Part print with two shaded views. Sizes in mm from the minimum x, y, z corner. A direction names the side the tool comes from. Round coordinates to 2 decimals unless told otherwise and drop trailing zeros. Order: outer loops, then holes, each group sorted by start corner. A loop starts at its lowest first (then second) coordinate and runs counter-clockwise, first axis right, second up. Notation, with made-up numbers: M 73,64.25 L 110,64.25 A17 ccw 110,81.25 Z; hole C -23.5,72 d2. An arc over 180 degrees is marked long. Answer as a JSON object with one key per item and string values.
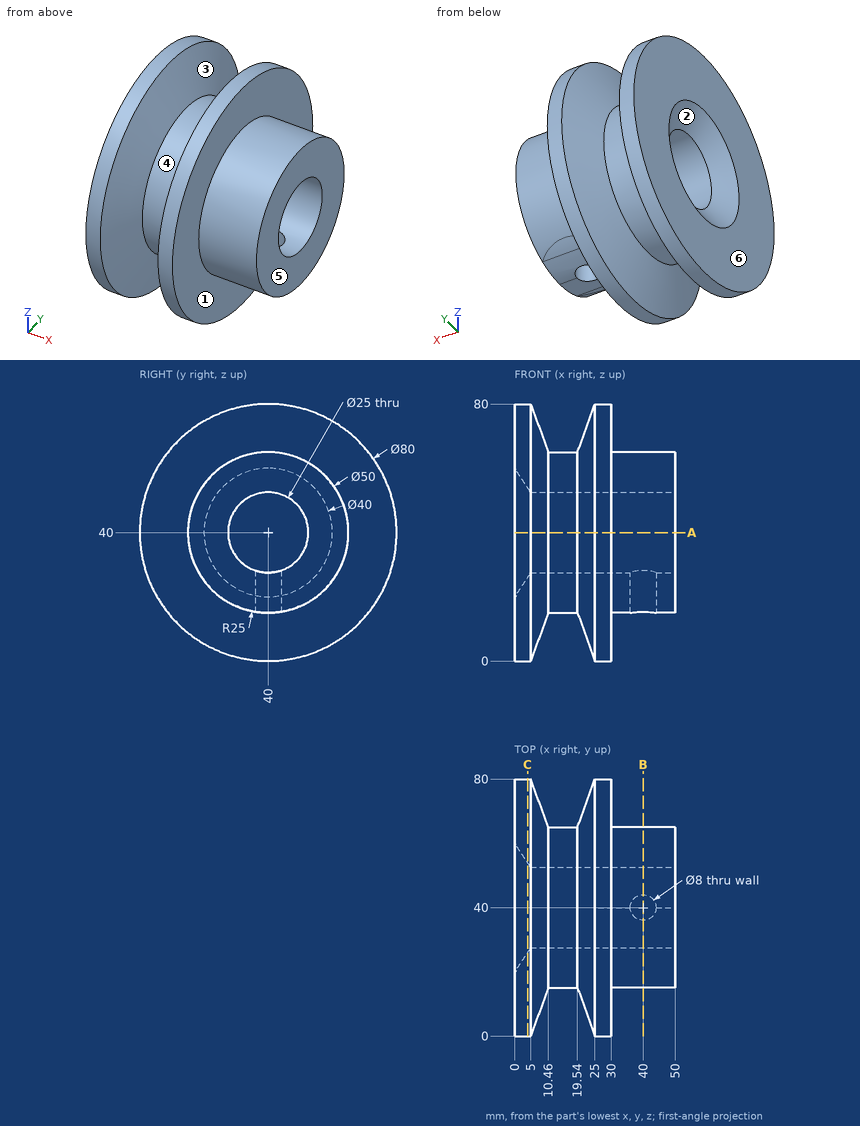
Item 1: Two-plate mould, pull along X, no slides. Class the marked faces 4, 5 and 6: released by +X, released by -X, zero draft, split by the parting line, or undercut.
Worked answers:
{"face 4": "undercut", "face 5": "released by +X", "face 6": "released by -X"}
Item 2: Saw through at A-A on z = 40. List the corners of the cut face in (x, y).
Worked answers:
{"outline": "M 0,0 L 5,0 L 10.46,15 L 19.54,15 L 25,0 L 30,0 L 30,15 L 50,15 L 50,27.5 L 5,27.5 L 0,20 Z; M 0,60 L 5,52.5 L 50,52.5 L 50,65 L 30,65 L 30,80 L 25,80 L 19.54,65 L 10.46,65 L 5,80 L 0,80 Z"}
Item 3: Saw through at C-C on x = 4. List the corners of the cut face in (y, z).
Worked answers:
{"outline": "C 40,40 d80; hole C 40,40 d28"}
Item 4: Drop flat-ended pins along their axis: pin 1 Ø5 at (x, z) = (25.5, 52) entering from -Y (1 decimal); pin 2 Ø2 at (x, y) = (37, 46) entering from -Z (1 decimal); pin 3 Ø2 at (x, y) = (32, 47) entering from +Z; pin 4 Ø20 at (y, z) = (40, 40) entering from +X. Give the stop position or say it passes through.
Worked answers:
{"pin 1": "stops at y = 1.1", "pin 2": "stops at z = 15.5", "pin 3": "stops at z = 64.27", "pin 4": "passes through"}
Item 5: Wall check: line 1 along Z through (x, y) = (19, 40); line 2 along Y through (x, z) = (40, 25). Give the ranges that are in metal, low to high. Write a range as [from, to].
Worked answers:
{"line 1": "z = [15, 27.5], [52.5, 65]", "line 2": "y = [20, 36], [44, 60]"}
Item 6: Saw through at B-B on x = 40. List the corners of the cut face in (y, z), and give its area (3 significant figures).
Worked answers:
{"outline": "M 36,15.32 L 36,28.16 A12.5 cw long 44,28.16 L 44,15.32 A25 ccw long Z", "area": "1,370 mm2"}
Item 7: 3-axis set-ups, long thin cutter, end or side, ignore diameter. For the marked faces 1, 2 and 3: which of +Z, -Z, +X, -X, +Y, -Y reach the whole face in a straight line?
Worked answers:
{"face 1": "+X", "face 2": "-X", "face 3": "none"}
